Geometry check sheet. Reference: the model listing, model coordinates, mm. Face numbers are marked on the shaded views. A direction names the side the tool comes from. Round coordinates to 2 decimals unless told otherwise and drop trailing zeros. Order: outer loops, then holes, each group sorted by start corner. A loop starts at its lowest first (then second) coordinate and runs counter-clockwise, first axis right, second up. Notation, with made-up numbers: (75.5, -13) - (83.5, -13) arc R22 ccw to (83.5, 0) - close; hole circle Ø7 at (73.5, 41.5). An arc over 180 degrees is marked (long way). Use a Markdown table: item, result. Add a question column.
(1) Mould release check, pull along X, two halves, no side actions. Record for the marked faces 3, 4 and 5: released by +X, released by -X, zero draft, split by the parting line, or undercut.
(2) Section check A-A on x = 15. Record the boundary of the cut face in (y, z), then the cut area to 3 significant figures.
(3) Section check B-B on x = 54.5. Record the boundary of the cut face in (y, z).
(4) Access from +Z, -Z, +X, -X, +Y, -Y to the whole of each face (thin tool, end or side, straight path). Record for the marked faces 1 and 2.
(5) Gauge pin test, flat ends, axial feed: P1, Ø1, axis at x = 58, z = 5.5, coming from the +Y side; P2, Ø1, axis at x = 21, y = 12, coming from the +Z side; P3, Ø4, axis at x = 31.5, y = -11, coming from the -Z side. Record the tip position at first contact, or that the pin passes through.
(6) Thickness scan on line 1 along Y through (x, z) = (104, 0); line 2 along Y through (x, z) = (102.1, 0); line 3 along X through (y, z) = (-4, -15). Record the ranges inside material, lowest first. Write a range as [from, to].
```python
from build123d import *

# Parameters (mm, degrees)
ESQUISSE1_W                      = 105
ESQUISSE1_H                      = 18
ENL_V_MAT_EXTRU_1_DEPTH          = 30
EXTRUSION1_START                 = 30
EXTRUSION1_DEPTH                 = 30
ESQUISSE5_W                      = 7
ESQUISSE5_H                      = 14
DIAM_TRE_DU_PER_AGE_M14_0_14_2_D = 14


with BuildPart() as part:
    # Esquisse1 → Révolution1 (revolve)
    with BuildSketch(Plane.XY, mode=Mode.PRIVATE) as r_volution1_sk:
        with Locations((52.5, 9)):
            Rectangle(ESQUISSE1_W, ESQUISSE1_H)
    revolve(r_volution1_sk.sketch.rotate(Axis((0, 0, 0), (1, 0, 0)), 270), axis=Axis((0, 0, 0), (1, 0, 0)))

    # Esquisse2 → Enlèv. mat.-Extru.1 (cut)
    with BuildSketch(Plane.ZY):
        with BuildLine():
            Line((-4, 17.549928775), (-4, -17.549928775))
            ThreePointArc((-4, -17.549928775), (18, 0), (-4, 17.549928775))
        make_face()
    extrude(amount=-ENL_V_MAT_EXTRU_1_DEPTH, mode=Mode.SUBTRACT)

    # Esquisse3 → Extrusion1 (add)
    with BuildSketch(Plane.ZY.offset(-30).offset(EXTRUSION1_START)):
        with BuildLine():
            Line((4, -17.549928775), (4, 17.549928775))
            ThreePointArc((4, 17.549928775), (18, 0), (4, -17.549928775))
        make_face()
    extrude(amount=-EXTRUSION1_DEPTH)

    # Esquisse4 → Enlèvement de matière-Révolution1 (revolve, cut)
    with BuildSketch(Plane(origin=(0, 0, 0), x_dir=(-1, 0, 0), z_dir=(0, 0, -1)), mode=Mode.PRIVATE) as enl_vement_de_mati_re_r_volution1_sk:
        Polygon((-105, 15), (-105, 0), (-90.339745962, 0), (-99, 15), (-101, 15), (-101, 17), (-103, 17), (-103, 15), align=None)
    revolve(enl_vement_de_mati_re_r_volution1_sk.sketch.rotate(Axis((105.000025, 0, 0), (-1, 0, 0)), 270), axis=Axis((105.000025, 0, 0), (-1, 0, 0)), mode=Mode.SUBTRACT)

    # Esquisse5 → Diamètre du perçage M14.0 (14)1 (revolve, cut)
    with BuildSketch(Plane(origin=(15, 0, 4), x_dir=(0, 1, 0), z_dir=(1, 0, 0))):
        with Locations((3.5, 7)):
            Rectangle(ESQUISSE5_W, ESQUISSE5_H)
    revolve(axis=Axis((15, 0, -2.35), (0, 0, 1)), mode=Mode.SUBTRACT)

    # Diamètre du perçage M14.0 (14)2 (through all)
    with Locations(Plane.XY.offset(-4)):
        with Locations((15, 0)):
            Hole(DIAM_TRE_DU_PER_AGE_M14_0_14_2_D / 2)


solid = part.part
```
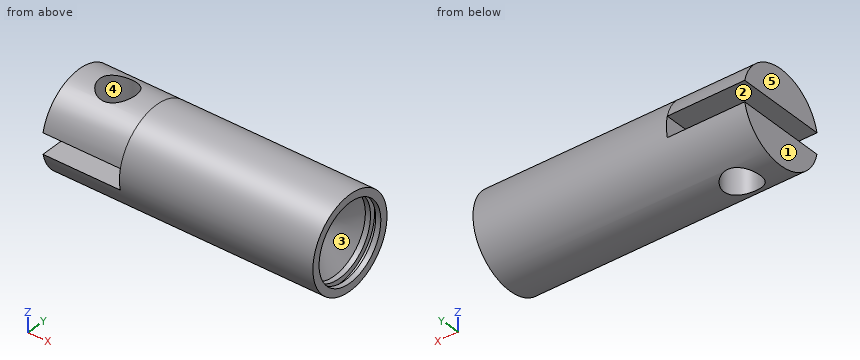
Check sheet entries:
| question | item | result |
|---|---|---|
| 1 | face 3 | released by +X |
| 1 | face 4 | undercut |
| 1 | face 5 | released by -X |
| 2 | outline | (-17.55, -4) arc R18 ccw to (-7, -16.58) - (-7, -4) - close; (-17.55, 4) - (-7, 4) - (-7, 16.58) arc R18 ccw to start; (7, -16.58) arc R18 ccw to (17.55, -4) - (7, -4) - close; (7, 4) - (17.55, 4) arc R18 ccw to (7, 16.58) - close |
| 2 | area | 353 mm2 |
| 3 | outline | circle Ø36 at (0, 0) |
| 4 | face 1 | +Z, -Z, -X, +Y, -Y |
| 4 | face 2 | -X, +Y, -Y |
| 5 | P1 | stops at y = 17.29 |
| 5 | P2 | stops at z = 13.85 |
| 5 | P3 | stops at z = -15.59 |
| 6 | line 1 | y = [-18, -15], [15, 18] |
| 6 | line 2 | y = [-18, -17], [17, 18] |
| 6 | line 3 | x = [0, 9.26], [20.74, 101], [103, 105] |
